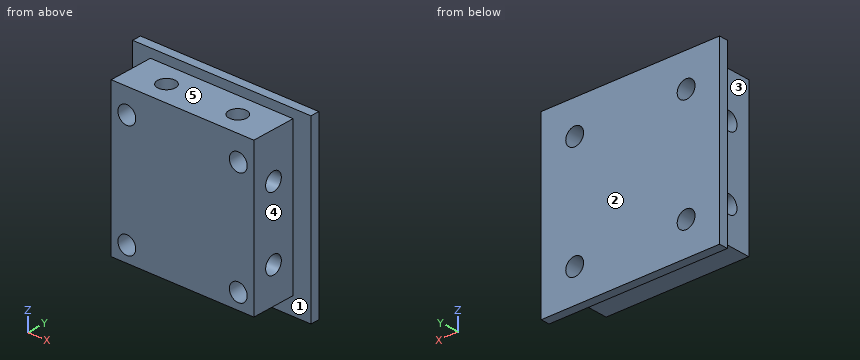
from build123d import *

# Parameters (mm, degrees)
SKETCH032_W     = 40
SKETCH032_H     = 40
SKETCH032_R     = 2
PAD018_DEPTH    = 2
SKETCH033_W     = 32
SKETCH033_H     = 34
SKETCH033_R     = 2
PAD019_DEPTH    = 10
SKETCH034_R     = 2
POCKET013_DEPTH = 8
SKETCH035_R     = 2
POCKET014_DEPTH = 8
SKETCH039_R     = 2
POCKET015_DEPTH = 8


with BuildPart() as part:
    # Sketch032 → Pad018 (new body)
    with BuildSketch(Plane.XZ):
        with Locations((0, 20)):
            Rectangle(SKETCH032_W, SKETCH032_H)
        with Locations((-12.5, 7.5)):
            Circle(SKETCH032_R, mode=Mode.SUBTRACT)
        with Locations((-12.5, 32.5)):
            Circle(SKETCH032_R, mode=Mode.SUBTRACT)
        with Locations((12.5, 32.5)):
            Circle(SKETCH032_R, mode=Mode.SUBTRACT)
        with Locations((12.5, 7.5)):
            Circle(SKETCH032_R, mode=Mode.SUBTRACT)
    extrude(amount=-PAD018_DEPTH)

    # Sketch033 (on Face9 of Pad018) → Pad019 (join)
    with BuildSketch(Plane.XZ):
        with Locations((0, 21)):
            Rectangle(SKETCH033_W, SKETCH033_H)
        with Locations((-12.5, 32.5)):
            Circle(SKETCH033_R, mode=Mode.SUBTRACT)
        with Locations((12.5, 32.5)):
            Circle(SKETCH033_R, mode=Mode.SUBTRACT)
        with Locations((-12.5, 7.5)):
            Circle(SKETCH033_R, mode=Mode.SUBTRACT)
        with Locations((12.5, 7.5)):
            Circle(SKETCH033_R, mode=Mode.SUBTRACT)
    extrude(amount=PAD019_DEPTH)

    # Sketch034 (on Face10 of Pad019) → Pocket013 (cut)
    with BuildSketch(Plane(origin=(-16, 0, 0), x_dir=(0, 0, -1), z_dir=(-1, 0, 0))):
        with Locations((-28, 5)):
            Circle(SKETCH034_R)
        with Locations((-12, 5)):
            Circle(SKETCH034_R)
    extrude(amount=-POCKET013_DEPTH, mode=Mode.SUBTRACT)

    # Sketch035 (on Face7 of Pocket013) → Pocket014 (cut)
    with BuildSketch(Plane(origin=(0, 0, 38), x_dir=(-1, 0, 0), z_dir=(0, 0, 1))):
        with Locations((-8, 5)):
            Circle(SKETCH035_R)
        with Locations((8, 5)):
            Circle(SKETCH035_R)
    extrude(amount=-POCKET014_DEPTH, mode=Mode.SUBTRACT)

    # Sketch039 (on Face8 of Pocket014) → Pocket015 (cut)
    with BuildSketch(Plane(origin=(16, 0, 0), x_dir=(0, 0, 1), z_dir=(1, 0, 0))):
        with Locations((12, 5)):
            Circle(SKETCH039_R)
        with Locations((28, 5)):
            Circle(SKETCH039_R)
    extrude(amount=-POCKET015_DEPTH, mode=Mode.SUBTRACT)


solid = part.part
Design review of the part built by this model. Coordinates are the model's own, in mm. Face numbers are marked on the shaded views. A direction names the side the tool comes from. Give positions to 0.01 mm unless a question says otherwise; leave off trailing zeros. Loops run counter-clockwise (first coordinate to the right, second up) from the corner with the lowest first, then second, coordinate; pieces in that order, holes last. Notation, with made-up numbers: M 19.5,59.5 L 75.5,59.5 A9 ccw 75.5,65.5 Z; hole C 43,62.5 d7. An arc over 180 degrees is marked long. Answer as a JSON object with one key per item and string values.
Item 1: We need section A-A (x = -12.5). State the section outline as (y, z) points, and give its area (3 significant figures).
Output values:
{"outline": "M -10,4 L 0,4 L 0,0 L 2,0 L 2,5.5 L -10,5.5 Z; M -10,9.5 L 2,9.5 L 2,30.5 L -10,30.5 Z; M -10,34.5 L 2,34.5 L 2,40 L 0,40 L 0,38 L -10,38 Z; hole C -5,12 d4; hole C -5,28 d4", "area": "299 mm2"}
Item 2: Wall thickness on line 1 along Z through (x, y) = (-12.5, -1); line 2 along X through (y, z) = (-6.75, 32); line 3 along Z through (x, y) = (12, -6): over which ranges is each line inside the solid? List them lowest first.
Output values:
{"line 1": "z = 4 to 5.5, 9.5 to 30.5, 34.5 to 38", "line 2": "x = -16 to -14.44, -10.56 to -8.97, -7.03 to 7.03, 8.97 to 10.56, 14.44 to 16", "line 3": "z = 4 to 5.56, 9.44 to 10.27, 13.73 to 26.27, 29.73 to 30.56, 34.44 to 38"}
Item 3: Machinability: for the marked faces 1, 2, 3, 4 and 5, which of the approach directions +Z, -Z, +X, -X, +Y, -Y give a long, thin tool a straight path to every point of the face, cutting with its end or side? Answer none if there is none.
Output values:
{"face 1": "-Y", "face 2": "+Z, -Z, +X, -X, +Y", "face 3": "+Z, -Z, -X, -Y", "face 4": "+Z, -Z, +X, -Y", "face 5": "+Z, +X, -X, -Y"}
Item 4: We need section B-B (y = -7.75). State the section outline as (x, z) points, and give its area (3 significant figures).
Output values:
{"outline": "M -16,4 L 16,4 L 16,38 L -16,38 Z; hole C -12.5,7.5 d4; hole C -12.5,32.5 d4; hole C 12.5,7.5 d4; hole C 12.5,32.5 d4", "area": "1,040 mm2"}
Item 5: We need section D-D (z = 28). State the section outline as (x, y) points, and give its area (3 significant figures).
Output values:
{"outline": "M -20,0 L -16,0 L -16,-3 L -8,-3 L -8,-7 L -16,-7 L -16,-10 L 16,-10 L 16,-7 L 8,-7 L 8,-3 L 16,-3 L 16,0 L 20,0 L 20,2 L -20,2 Z", "area": "336 mm2"}
Item 6: For P1, Ø3, axis at y = -5.5, z = 13, coming from the +X side; P2, Ø6, axis at x = 11, y = -8, coming from the -Z side; P3, Ø4.5, axis at y = -5.5, z = 27.5, coming from the -X side, all flat-tipped, find the tip position at first contact; note any pin that passes through.
Output values:
{"P1": "stops at x = 16", "P2": "stops at z = 4", "P3": "stops at x = -16"}
